Solid Edge part; units mm, degrees
sketch "Sketch1" plane through (0, 0, 0) normal (0, -1, 0) x (1, 0, 0)
  circle A0 centre (0, 0) radius 5.9
extrude "Protrusion1" add sketch "Sketch1" against normal blind 2.54
sketch "Sketch2" plane through (0, 2.54, 0) normal (0, 1, 0) x (0, 0, -1)
  circle A0 centre (0, 0) radius 6.25
extrude "Ajout_matière_3" add sketch "Sketch2" along normal blind 14.6
fillet "Congé_1" radius 0.5 1 edges at (-5.9, 0, 0)
fillet "Congé_2" radius 0.2 1 edges at (0, 2.54, 6.25)
chamfer "Chanfrein_1" distance 1 angle 86 1 edges at (0, 17.14, 6.25) measured on face at (-4.0417, 17.14, -4.2917)
sketch "Sketch3" plane through (0, 17.14, 0) normal (0, 1, 0) x (1, 0, 0)
  circle A0 centre (0, 0) radius 3.25
extrude "Enlèvement_matière_1" cut sketch "Sketch3" against normal blind 26
sketch "Sketch4" plane through (0, 17.14, 0) normal (0, 1, 0) x (1, 0, 0)
  circle A0 centre (0, -6.25) radius 1.75
  circle A1 centre (-4.4179, -4.4209) radius 1.75
  circle A2 centre (-6.25, 0) radius 1.75
  circle A3 centre (-4.4179, 4.4209) radius 1.75
  circle A4 centre (0, 6.25) radius 1.75
  circle A5 centre (4.4179, 4.4209) radius 1.75
  circle A6 centre (6.25, 0) radius 1.75
  circle A7 centre (4.397, -4.4417) radius 1.75
extrude "Enlèvement_matière_3" cut sketch "Sketch4" against normal blind 8
Input: part model. Units: mm. Frame: model coordinates. A direction names the side the tool comes from. Give positions to 0.01 mm unless a question says otherwise; leave off trailing zeros. Write each loop counter-clockwise with the first axis right and the second up, starting at its lowest first coordinate (ties: lowest second). Pieces come first, ordered by that corner, then holes. Notation, with made-up numbers: (53, 25) - (82, 25) arc R30 cw to (82, 47) - close; hole circle Ø3 at (-13, 21.5). An arc over 180 degrees is marked (long way). Write item = value, one per line. Start each with the question number.
1. Section query A-A, the plane x = 0. Output: boundary loops of the cut face in (y, z).
2. Access query for faces 1 (the cylindrical face through (3.161, 13.196, -3.204)), 2 (the cylindrical face through (-5.894, 1.506, 0.259)), 3 (the cylindrical face through (0, 13.2, -4.5)). Directions: +Z, -Z, +X, -X, +Y, -Y. A direction counts if a zero-diameter tool reaches every point of the face in a straight line with its end or side. Return the directions, or none.
3. Section query B-B, the plane z = 0. Output: boundary loops of the cut face in (x, y), then the cut area to 3 significant figures.
4. First-contact query: pin 1 Ø1.2 at (x, z) = (4, 4) entering from +Y; pin 2 Ø4 at (y, z) = (3.5, 3) entering from +X; pin 3 Ø4 at (x, z) = (0, 0) entering from -Y; pin 4 Ø2 at (y, z) = (6, 1.5) entering from -X. Flat tips, straight axial feed; report the tip coordinate or a pass-through.
5. Section query C-C, the plane y = 13.25. Output: boundary loops of the cut face in (x, z).
6. Section query D-D, the plane y = 4.5. Output: boundary loops of the cut face in (x, z).
7. Ray query, L1, parallel to Z at x = 0, y = 10.25; L2, parallel to X at y = 1.75, z = -3. Return the intervals inside material, ascending.
Check sheet entries:
q1.outline = (0, -5.4) arc R0.5 ccw to (0.5, -5.9) - (2.54, -5.9) - (2.54, -6.05) arc R0.2 ccw to (2.74, -6.25) - (2.84, -6.25) - (9.14, -5.81) - (9.14, -4.5) - (17.14, -4.5) - (17.14, -3.25) - (0, -3.25) - close; (0, 3.25) - (17.14, 3.25) - (17.14, 4.5) - (9.14, 4.5) - (9.14, 5.81) - (2.84, 6.25) - (2.74, 6.25) arc R0.2 ccw to (2.54, 6.05) - (2.54, 5.9) - (0.5, 5.9) arc R0.5 ccw to (0, 5.4) - close
q2.face_1 = +Y
q2.face_2 = -Y
q2.face_3 = -Z, +Y
q3.outline = (-6.25, 2.74) arc R0.2 ccw to (-6.05, 2.54) - (-5.9, 2.54) - (-5.9, 0.5) arc R0.5 ccw to (-5.4, 0) - (-3.25, 0) - (-3.25, 17.14) - (-4.5, 17.14) - (-4.5, 9.14) - (-5.81, 9.14) - (-6.25, 2.84) - close; (3.25, 0) - (5.4, 0) arc R0.5 ccw to (5.9, 0.5) - (5.9, 2.54) - (6.05, 2.54) arc R0.2 ccw to (6.25, 2.74) - (6.25, 2.84) - (5.81, 9.14) - (4.5, 9.14) - (4.5, 17.14) - (3.25, 17.14) - close
q3.area = 70.2 mm2
q4.pin_1 = 9.14
q4.pin_2 = 6.15
q4.pin_3 = through
q4.pin_4 = -6.03
q5.outline = (-5.32, -1.48) arc R5.52 ccw to (-4.81, -2.72) arc R1.75 cw to (-2.71, -4.81) arc R5.52 ccw to (-1.48, -5.32) arc R1.75 cw to (1.48, -5.32) arc R5.52 ccw to (2.71, -4.81) arc R1.75 cw to (4.81, -2.72) arc R5.52 ccw to (5.32, -1.48) arc R1.75 cw to (5.32, 1.48) arc R5.52 ccw to (4.8, 2.74) arc R1.75 cw to (2.69, 4.82) arc R5.52 ccw to (1.48, 5.32) arc R1.75 cw to (-1.48, 5.32) arc R5.52 ccw to (-2.71, 4.81) arc R1.75 cw to (-4.81, 2.72) arc R5.52 ccw to (-5.32, 1.48) arc R1.75 cw to start; hole circle Ø6.5 at (0, 0)
q6.outline = circle Ø12.27 at (0, 0); hole circle Ø6.5 at (0, 0)
q7.L1 = -4.5 to -3.25, 3.25 to 4.5
q7.L2 = -5.08 to -1.25, 1.25 to 5.08
